from build123d import *

# Parameters (mm, degrees)
SKETCH1_W               = 20
SKETCH1_H               = 25
BOSS_EXTRUDE1_DEPTH     = 17
CUT_EXTRUDE1_DEPTH      = 32.843366656
BOSS_EXTRUDE2_DEPTH     = 5
SKETCH4_R               = 2
CUT_EXTRUDE2_DEPTH      = 37.249137921
SKETCH6_W               = 20
SKETCH6_H               = 20
BOSS_EXTRUDE3_DEPTH     = 7
SKETCH8_W               = 8.2
SKETCH8_H               = 3.8
CUT_EXTRUDE3_DEPTH      = 41.401113846
CUT_EXTRUDE4_REACH      = 43.379
CUT_EXTRUDE4_END_RADIUS = 7
SKETCH7_R               = 2
SKETCH9_W               = 15
SKETCH9_H               = 7.5
CUT_EXTRUDE5_DEPTH      = 2
SKETCH10_W              = 10
SKETCH10_H              = 0.75
CUT_EXTRUDE6_DEPTH      = 41.01249811
CUT_EXTRUDE7_START      = 20
SKETCH9_2_W             = 15
SKETCH9_2_H             = 7.5
CUT_EXTRUDE7_DEPTH      = 2.5


with BuildPart() as part:
    # Sketch1 → Boss-Extrude1 (new body)
    with BuildSketch(Plane(origin=(0, 0, 0), x_dir=(1, 0, 0), z_dir=(0, 1, 0))):
        Rectangle(SKETCH1_W, SKETCH1_H)
    extrude(amount=BOSS_EXTRUDE1_DEPTH)

    # Sketch2 → Cut-Extrude1 (cut, through all)
    with BuildSketch(Plane.XY.offset(12.5)):
        with BuildLine():
            Line((0, 2), (-6.062177826, 5.5))
            ThreePointArc((-6.062177826, 5.5), (0, 16), (6.062177826, 5.5))
            Line((6.062177826, 5.5), (0, 2))
        make_face()
    extrude(amount=-CUT_EXTRUDE1_DEPTH, mode=Mode.SUBTRACT)

    # Sketch3 → Boss-Extrude2 (add)
    with BuildSketch(Plane.XY.offset(12.5)):
        Polygon((10, 0), (20, 0), (20, -10), (-20, -10), (-20, 0), (-10, 0), align=None)
    boss_extrude2 = extrude(amount=-BOSS_EXTRUDE2_DEPTH)

    # Mirror1: Boss-Extrude2 across plane
    add(boss_extrude2.mirror(Plane.XY))

    # Sketch4 → Cut-Extrude2 (cut, through all)
    with BuildSketch(Plane.XY.offset(12.5)):
        with Locations((16, -5)):
            Circle(SKETCH4_R)
        with Locations((-16, -5)):
            Circle(SKETCH4_R)
    extrude(amount=-CUT_EXTRUDE2_DEPTH, mode=Mode.SUBTRACT)

    # Sketch6 → Boss-Extrude3 (add)
    with BuildSketch(Plane(origin=(0, 17, 0), x_dir=(1, 0, 0), z_dir=(0, 1, 0))):
        Rectangle(SKETCH6_W, SKETCH6_H)
    extrude(amount=BOSS_EXTRUDE3_DEPTH)

    # Sketch8 → Cut-Extrude3 (cut, through all)
    with BuildSketch(Plane(origin=(10, 0, 0), x_dir=(0, 0, -1), z_dir=(1, 0, 0))):
        with Locations((0, 18.9)):
            Rectangle(SKETCH8_W, SKETCH8_H)
    extrude(amount=-CUT_EXTRUDE3_DEPTH, mode=Mode.SUBTRACT)

    # Cut-Extrude4: up to this cylinder (the profile starts outside it)
    cut_extrude4_end = Plane(origin=(0, 9, 0), z_dir=(0, 0, 1)) * Cylinder(CUT_EXTRUDE4_END_RADIUS, 101.758, mode=Mode.PRIVATE)
    # Sketch7 → Cut-Extrude4 (cut, up to the surface)
    with BuildSketch(Plane(origin=(0, 24, 0), x_dir=(1, 0, 0), z_dir=(0, 1, 0)), mode=Mode.PRIVATE) as cut_extrude4_sk1:
        with Locations(Location((0, 0, 0), (0, 0, 270))):
            Circle(SKETCH7_R)
    cut_extrude4_tool1 = extrude(cut_extrude4_sk1.sketch, amount=-CUT_EXTRUDE4_REACH, mode=Mode.PRIVATE) - cut_extrude4_end
    add(cut_extrude4_tool1.solids().sort_by_distance((0, 24, 0))[0], mode=Mode.SUBTRACT)

    # Sketch9 → Cut-Extrude5 (cut)
    with BuildSketch(Plane.ZY.offset(-10)):
        with Locations((0, 3.75)):
            Rectangle(SKETCH9_W, SKETCH9_H)
    extrude(amount=CUT_EXTRUDE5_DEPTH, mode=Mode.SUBTRACT)

    # Sketch10 → Cut-Extrude6 (cut, through all)
    with BuildSketch(Plane.XY.offset(12.5)):
        with Locations((-15, -5)):
            Rectangle(SKETCH10_W, SKETCH10_H)
        with Locations((15, -5)):
            Rectangle(SKETCH10_W, SKETCH10_H)
    extrude(amount=-CUT_EXTRUDE6_DEPTH, mode=Mode.SUBTRACT)

    # Sketch9<2> → Cut-Extrude7 (cut)
    with BuildSketch(Plane.ZY.offset(-10).offset(CUT_EXTRUDE7_START)):
        with Locations((0, 3.75)):
            Rectangle(SKETCH9_2_W, SKETCH9_2_H)
    extrude(amount=-CUT_EXTRUDE7_DEPTH, mode=Mode.SUBTRACT)


solid = part.part
Input: part model. Units: mm. Frame: model coordinates. A direction names the side the tool comes from. Coordinates: 2 decimals unless noted, no trailing zeros. Order: outer loops, then holes, each group sorted by start corner. A loop starts at its lowest first (then second) coordinate and runs counter-clockwise, first axis right, second up. Notation, with made-up numbers: M 47.25,23.25 L 56.25,23.25 A10 ccw 56.25,38.25 Z; hole C -8,46 d10. An arc over 180 degrees is marked long. Write item = value, one per line. Start each with the question number.
(1) Section B-B on y = 9. Output: boundary loops of the cut face in (x, z), and give its area (3 significant figures).
(2) Section A-A on z = -3. Output: boundary loops of the cut face in (x, y), and give its area (3 significant figures).
(3) Section C-C on z = 10.75. Output: boundary loops of the cut face in (x, y) (3 decimals), and give its area (3 significant figures).
(4) First-contact query: P1, Ø0.8, axis at x = -1.5, z = -11.5, coming from the +Y side; P2, Ø2, axis at y = 3.5, z = 1.5, coming from the -X side; P3, Ø5.5, axis at x = 0, y = 22, coming from the -Z side. Flat tips, straight axial feed; report the tip coordinate or a pass-through.
(5) Section D-D on x = -9. Output: boundary loops of the cut face in (y, z), and give its area (3 significant figures).
(6) Line query: line 1 along Y through (x, z) = (0, -3.25); line 2 along X through (y, z) = (16.2, 0); line 3 along X through (y, z) = (-4, -8.25). Output: solid intervals per line, ascending. Write a range as [from, to].
(7) Pull-direction query (Z, two-part tool) for faces 6 (the cylindrical face through (-2, 22, 0)), 7 (the flat face through (0, 20, -10)), 8 (the flat face through (-12, -5.375, -10)); classes: released by +Z, released by -Z, zero draft, split by the parting line, or undercut.
(8) Reachability of faces 1 (the flat face through (0, 20, 10)), 2 (the flat face through (-19, -4.625, -10)), 3 (the flat face through (12, -5.375, 10)), 4 (the cylindrical face through (-16, -7, -10)), 5 (the flat face through (-15, 0, -10)) from +Z, -Z, +X, -X, +Y, -Y: full face, straight path, thin tool, end or side. Return the list, or none.
Result set:
q1.outline = M -10,-12.5 L -7,-12.5 L -7,12.5 L -10,12.5 Z; M 7,-12.5 L 10,-12.5 L 10,12.5 L 7,12.5 Z
q1.area = 150 mm²
q2.outline = M -10,7.5 L -7.5,7.5 L -7.5,0 L 8,0 L 8,7.5 L 10,7.5 L 10,17 L -10,17 Z; M -10,20.8 L 10,20.8 L 10,24 L -10,24 Z; hole M -6.06,5.5 L 0,2 L 6.06,5.5 A7 ccw long Z
q2.area = 225 mm²
q3.outline = M -20,-10 L 20,-10 L 20,-5.375 L 17.965,-5.375 A2 cw 14.035,-5.375 L 10,-5.375 L 10,-4.625 L 14.035,-4.625 A2 cw 17.965,-4.625 L 20,-4.625 L 20,0 L 10,0 L 10,17 L -10,17 L -10,0 L -20,0 L -20,-4.625 L -17.965,-4.625 A2 cw -14.035,-4.625 L -10,-4.625 L -10,-5.375 L -14.035,-5.375 A2 cw -17.965,-5.375 L -20,-5.375 Z; hole M -6.062,5.5 L 0,2 L 6.062,5.5 A7 ccw long Z
q3.area = 561 mm²
q4.P1 = 17
q4.P2 = -7.5
q4.P3 = -10
q5.outline = M -10,-12.5 L 17,-12.5 L 17,-10 L 24,-10 L 24,10 L 17,10 L 17,12.5 L -10,12.5 L -10,7.5 L 7.5,7.5 L 7.5,-7.5 L -10,-7.5 Z; hole M 17,-4.1 L 20.8,-4.1 L 20.8,4.1 L 17,4.1 Z
q5.area = 521 mm²
q6.line_1 = [0, 2], [16, 17], [20.8, 24]
q6.line_2 = [-10, -2], [2, 10]
q6.line_3 = [-20, -17.73], [-14.27, 14.27], [17.73, 20]
q7.face_6 = undercut
q7.face_7 = released by -Z
q7.face_8 = zero draft
q8.face_1 = +Z, +X, -X, +Y
q8.face_2 = +Z, -Z, -X
q8.face_3 = +Z, -Z, +X
q8.face_4 = +Z, -Z
q8.face_5 = +Z, -Z, -X, +Y
